Work out the finished part from the listing and answer in its coordinate system (mm). Face numbers are marked on the shaded views. A direction names the side the tool comes from. Give positions to 0.01 mm unless a question says otherwise; leave off trailing zeros. Loops run counter-clockwise (first coordinate to the right, second up) from the corner with the lowest first, then second, coordinate; pieces in that order, holes last. Notation, with made-up numbers: (8.5, -3) - (35.5, -3) arc R24 ccw to (35.5, 24) - close; hole circle Ø1 at (-14.75, 59). An arc over 180 degrees is marked (long way). One line per item, written item: value.
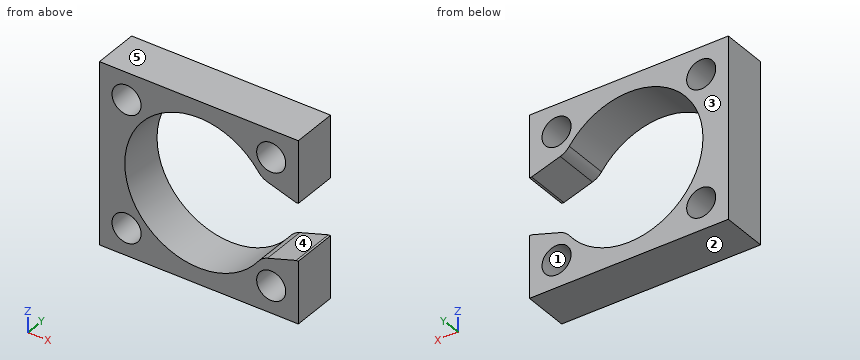
from build123d import *

# Parameters (mm, degrees)
SKETCH1_W              = 34.925
SKETCH1_H              = 31.75
PLATE_DEPTH            = 4
F_10_CLEARANCE_HOLE1_D = 5.1054
LOAD_CELL_CUTOUT_REACH = 26.919
FILLET1_R              = 3.175


with BuildPart() as part:
    # Sketch1 → Plate (new, symmetric)
    with BuildSketch(Plane(origin=(0, 0, 0), x_dir=(1, 0, 0), z_dir=(0, 1, 0))):
        Rectangle(SKETCH1_W, SKETCH1_H)
    extrude(amount=PLATE_DEPTH, both=True)

    # #10 Clearance Hole1 (through all)
    with Locations(Plane(origin=(0, 4, 0), x_dir=(1, 0, 0), z_dir=(0, 1, 0))):
        with Locations((-12.7, 11.1125), (12.7, 11.1125), (12.7, -11.1125), (-12.7, -11.1125)):
            Hole(F_10_CLEARANCE_HOLE1_D / 2)

    # Sketch4 → Load Cell Cutout (cut, up to next)
    with BuildSketch(Plane(origin=(0, 4, 0), x_dir=(1, 0, 0), z_dir=(0, 1, 0)), mode=Mode.PRIVATE) as load_cell_cutout_sk1:
        with BuildLine():
            Line((11.009869163, 6.927542495), (17.078427656, 5.008))
            Line((17.078427656, 5.008), (22.733, 5.008))
            Line((22.733, 5.008), (22.733, -5.008))
            Line((22.733, -5.008), (17.078427656, -5.008))
            Line((17.078427656, -5.008), (11.009869163, -6.927542495))
            ThreePointArc((11.009869163, -6.927542495), (-13.008, 0), (11.009869163, 6.927542495))
        make_face()
    load_cell_cutout_tool1 = extrude(load_cell_cutout_sk1.sketch, amount=-LOAD_CELL_CUTOUT_REACH, mode=Mode.PRIVATE) & part.part
    add(load_cell_cutout_tool1.solids().sort_by_distance((2.977457, 4, 0))[0], mode=Mode.SUBTRACT)

    # Fillet1
    fillet1_edges = [part.edges().sort_by_distance(p)[0] for p in [
        (11.009869163, 0, 6.927542495),
        (11.009869163, 0, -6.927542495),
    ]]
    fillet(fillet1_edges, radius=FILLET1_R)


solid = part.part
1. Section D-D (y = 1.75) is taken. Count the separate pieces of the cut face and the enclosed holes in it, and give its area (3 significant figures).
Output:
separate pieces: 1
enclosed holes: 4
area: 438 mm²
2. Section A-A (x = 13.5) is taken. Write down the section's boundary in (y, z) (3 decimals), and give its area (3 significant figures).
Output:
outline: (-4, -15.875) - (4, -15.875) - (4, -13.537) - (-4, -13.537) - close; (-4, -8.688) - (4, -8.688) - (4, -6.14) - (-4, -6.14) - close; (-4, 6.14) - (4, 6.14) - (4, 8.688) - (-4, 8.688) - close; (-4, 13.537) - (4, 13.537) - (4, 15.875) - (-4, 15.875) - close
area: 78.2 mm²
3. The mould has two halves that part along Z. Classify the marked faces 1, 2 and 3: released by +Z, released by -Z, zero draft, split by the parting line, or undercut.
Output:
face 1: undercut
face 2: released by -Z
face 3: zero draft
4. For the marked faces 4 and 5, determine the directions among +Z, -Z, +X, -X, +Y, -Y from which every point of the face is accessible in a straight line to the end or side of a thin tool.
Output:
face 4: +Y, -Y
face 5: +Z, +X, -X, +Y, -Y
5. Flat-ended cylindrical pins translate along their axes: pin 1 Ø3 at (y, z) = (2, 2) entering from +X; pin 2 Ø8 at (x, z) = (11, 5) entering from -Y; pin 3 Ø4 at (x, z) = (12.7, 11.11) entering from +Y. Find the tip coordinate at first contact, or state that the pin passes through.
Output:
pin 1: stops at x = -12.53
pin 2: stops at y = -4
pin 3: passes through
6. Section B-B (x = -8) is taken. Write down the section's boundary in (y, z) (3 decimals).
Output:
outline: (-4, -15.875) - (4, -15.875) - (4, -10.257) - (-4, -10.257) - close; (-4, 10.257) - (4, 10.257) - (4, 15.875) - (-4, 15.875) - close
7. Section C-C (z = 9) is taken. Write down the section's boundary in (x, y), and give its area (3 significant figures).
Output:
outline: (-17.46, -4) - (-14.13, -4) - (-14.13, 4) - (-17.46, 4) - close; (-11.27, -4) - (-9.39, -4) - (-9.39, 4) - (-11.27, 4) - close; (9.39, -4) - (11.27, -4) - (11.27, 4) - (9.39, 4) - close; (14.13, -4) - (17.46, -4) - (17.46, 4) - (14.13, 4) - close
area: 83.3 mm²
8. Find the intervals of material crossed by line 1 along X through (y, z) = (1.5, 11); line 2 along Z through (x, y) = (13, 0.75) (3 decimals); line 3 along X through (y, z) = (-1.75, -11.5), in increasing order.
Output:
line 1: x = -17.46 to -15.25, -10.15 to -6.94, 6.94 to 10.15, 15.25 to 17.46
line 2: z = -15.875 to -13.648, -8.577 to -6.298, 6.298 to 8.577, 13.648 to 15.875
line 3: x = -17.46 to -15.22, -10.18 to -6.08, 6.08 to 10.18, 15.22 to 17.46
